Read the model definition and answer for the solid it produces. Units are mm, in the model's axes. A direction names the side the tool comes from. Give positions to 0.01 mm unless a question says otherwise; leave off trailing zeros. Loops run counter-clockwise (first coordinate to the right, second up) from the corner with the lowest first, then second, coordinate; pieces in that order, holes last.
(1) Which of the six approach directions +Z, -Z, +X, -X, +Y, -Y give full straight-line access (tool end or side, diameter ignored) to faces 5 (the face through (28, -8, 2)), 6 (the face through (-17.034, -7.348, 9.691)), 7 (the face through (29, -29.583, 10))?
(2) Determine the mould class of faces 1 (the face through (66.391, 25.125, 9.691)), 2 (the face through (29, 26.842, 10)), 3 (the face through (20.6, -31.9, 17.6)), 4 (the face through (40.956, -36.022, 9.691)) for opening direction Y: pulls with the +Y half, pulls with the -Y half, needs draft (parallel to the pull), parting line crosses it, or undercut.
(3) Each of these flat-tipped pins is pushed along its axis until it touches: P1, Ø1.5, axis at y = -30, z = 10, coming from the +X side (3 decimals); P2, Ø4.5, axis at x = -3.5, y = -38, coming from the +Z side; P3, Ø0.8, axis at x = 31, y = -29, coming from the +Z side; P4, Ø3, axis at x = 50, z = 3, coming from the -Y side. Where does it stop, or does it pass through?
(4) Straight lines are drawn through the part: probe 1 along Y at (x, z) = (55, 17.25); probe 2 along X at (y, z) = (-1, 9.5); probe 3 along X at (y, z) = (1, 9.25). For each, find the intervals that lie inside material, in ascending order.
(5) Find section B-B, the plane z = 11.75. State how many separate pieces and enclosed holes the cut face has, then the cut area to 3 significant figures.
(6) Find section A-A, the plane x = 29. Write down the section's boundary in (y, z).
```python
from build123d import *

# Parameters (mm, degrees)
EXTRUDE_1_DEPTH                    = 2
EXTRUDE_2_DEPTH                    = 14
EXTRUDE_3_DEPTH                    = 15.6000508
FILLET_1_R                         = 2
SKETCH_12_W                        = 10.2
SKETCH_12_H                        = 1.9
USB_TYPEC_LOWER_HALF_OPENING_DEPTH = 4


with BuildPart() as part:
    # 草图1 → 凸台-拉伸1 (new body)
    with BuildSketch(Plane.XY):
        with BuildLine():
            Line((-18.736989068, -43.807492656), (7.319785463, -43.807492656))
            ThreePointArc((7.319785463, -43.807492656), (8.845661337, -43.503976443), (10.139236063, -42.639636403))
            Line((10.139236063, -42.639636403), (23.19168867, -29.587186336))
            ThreePointArc((23.19168867, -29.587186336), (23.195810689, -29.58443157), (23.200673199, -29.583464208))
            Line((23.200673199, -29.583464208), (34.512272144, -29.583464208))
            ThreePointArc((34.512272144, -29.583464208), (34.51713329, -29.584431533), (34.521254362, -29.587185298))
            Line((34.521254362, -29.587185298), (47.573709045, -42.639637441))
            ThreePointArc((47.573709045, -42.639637441), (48.867282822, -43.503976481), (50.393157333, -43.807492656))
            Line((50.393157333, -43.807492656), (75.552353414, -43.807492656))
            ThreePointArc((75.552353414, -43.807492656), (78.607819066, -42.38196989), (79.478533005, -39.124694535))
            Line((79.478533005, -39.124694535), (68.376081771, 23.550429382))
            ThreePointArc((68.376081771, 23.550429382), (67.011684276, 25.910401612), (64.449902577, 26.842240644))
            Line((64.449902577, 26.842240644), (-7.634537883, 26.842240644))
            ThreePointArc((-7.634537883, 26.842240644), (-10.196320099, 25.910401179), (-11.560717313, 23.550428053))
            Line((-11.560717313, 23.550428053), (-22.663168183, -39.124693813))
            ThreePointArc((-22.663168183, -39.124693813), (-21.792454719, -42.381969476), (-18.736989068, -43.807492656))
        make_face()
    extrude(amount=EXTRUDE_1_DEPTH)

    # 草图4 → 凸台-拉伸2 (add)
    # profile 1 of 4: a face of its own
    with BuildSketch(Plane.XY.offset(2)):
        with BuildLine():
            ThreePointArc((-5.872384963, -37.375183791), (-2.822381153, -40.425187601), (0.227622657, -37.375183791))
            ThreePointArc((0.227622657, -37.375183791), (-2.822381153, -34.325179981), (-5.872384963, -37.375183791))
        make_face()
        with BuildLine():
            ThreePointArc((-0.772377343, -37.375183791), (-2.822381153, -35.325179981), (-4.872384963, -37.375183791))
            ThreePointArc((-4.872384963, -37.375183791), (-2.822381153, -39.425187601), (-0.772377343, -37.375183791))
        make_face(mode=Mode.SUBTRACT)
    # profile 2 of 4: a face of its own
    with BuildSketch(Plane.XY.offset(2)):
        with BuildLine():
            ThreePointArc((56.727742037, -37.375183791), (59.777745847, -40.425187601), (62.827749657, -37.375183791))
            ThreePointArc((62.827749657, -37.375183791), (59.777745847, -34.325179981), (56.727742037, -37.375183791))
        make_face()
        with BuildLine():
            ThreePointArc((61.827749657, -37.375183791), (59.777745847, -35.325179981), (57.727742037, -37.375183791))
            ThreePointArc((57.727742037, -37.375183791), (59.777745847, -39.425187601), (61.827749657, -37.375183791))
        make_face(mode=Mode.SUBTRACT)
    # profile 3 of 4: a face of its own
    with BuildSketch(Plane.XY.offset(2)):
        with BuildLine():
            ThreePointArc((69.049761341, 9.106909173), (65.999757531, 12.156912983), (62.949753721, 9.106909173))
            ThreePointArc((62.949753721, 9.106909173), (65.999757531, 6.056905363), (69.049761341, 9.106909173))
        make_face()
        with BuildLine():
            ThreePointArc((63.949753721, 9.106909173), (65.999757531, 7.056905363), (68.049761341, 9.106909173))
            ThreePointArc((68.049761341, 9.106909173), (65.999757531, 11.156912983), (63.949753721, 9.106909173))
        make_face(mode=Mode.SUBTRACT)
    # profile 4 of 4: a face of its own
    with BuildSketch(Plane.XY.offset(2)):
        with BuildLine():
            ThreePointArc((-6.519385217, 1.613894187), (-3.469381407, -1.436109623), (-0.419377597, 1.613894187))
            ThreePointArc((-0.419377597, 1.613894187), (-3.469381407, 4.663897997), (-6.519385217, 1.613894187))
        make_face()
        with BuildLine():
            ThreePointArc((-1.419377597, 1.613894187), (-3.469381407, 3.663897997), (-5.519385217, 1.613894187))
            ThreePointArc((-5.519385217, 1.613894187), (-3.469381407, -0.436109623), (-1.419377597, 1.613894187))
        make_face(mode=Mode.SUBTRACT)
    extrude(amount=EXTRUDE_2_DEPTH)

    # 草图6 → 凸台-拉伸3 (add)
    with BuildSketch(Plane.XY.offset(2)):
        with BuildLine():
            Line((-11.560717313, 23.550428053), (-22.663168183, -39.124693813))
            ThreePointArc((-22.663168183, -39.124693813), (-21.792454719, -42.381969476), (-18.736989068, -43.807492656))
            Line((-18.736989068, -43.807492656), (7.319785463, -43.807492656))
            ThreePointArc((7.319785463, -43.807492656), (8.845661337, -43.503976443), (10.139236063, -42.639636403))
            Line((10.139236063, -42.639636403), (23.19168867, -29.587186337))
            ThreePointArc((23.19168867, -29.587186337), (23.195810689, -29.58443157), (23.200673199, -29.583464208))
            Line((23.200673199, -29.583464208), (34.512272144, -29.583464208))
            ThreePointArc((34.512272144, -29.583464208), (34.51713329, -29.584431533), (34.521254362, -29.587185298))
            Line((34.521254362, -29.587185298), (47.573709045, -42.639637441))
            ThreePointArc((47.573709045, -42.639637441), (48.867282822, -43.503976481), (50.393157333, -43.807492656))
            Line((50.393157333, -43.807492656), (75.552353414, -43.807492656))
            ThreePointArc((75.552353414, -43.807492656), (78.607819066, -42.38196989), (79.478533005, -39.124694535))
            Line((79.478533005, -39.124694535), (68.376081771, 23.550429382))
            ThreePointArc((68.376081771, 23.550429382), (67.011684276, 25.910401612), (64.449902577, 26.842240644))
            Line((64.449902577, 26.842240644), (-7.634537883, 26.842240644))
            ThreePointArc((-7.634537883, 26.842240644), (-10.196320099, 25.910401179), (-11.560717313, 23.550428053))
        make_face()
        with BuildLine():
            Line((-10.576047254, 23.376000774), (-21.678498124, -39.299121091))
            ThreePointArc((-21.678498124, -39.299121091), (-21.026156001, -41.739485021), (-18.736988894, -42.807492656))
            Line((-18.736988894, -42.807492656), (7.319785463, -42.807492656))
            ThreePointArc((7.319785463, -42.807492656), (8.462977611, -42.580097033), (9.432128831, -41.932530072))
            Line((9.432128831, -41.932530072), (22.484540842, -28.880120606))
            ThreePointArc((22.484540842, -28.880120606), (22.813100147, -28.660563268), (23.200672562, -28.583464208))
            Line((23.200672562, -28.583464208), (34.512322586, -28.58346421))
            ThreePointArc((34.512322586, -28.58346421), (34.899840317, -28.660561774), (35.228361593, -28.880078967))
            Line((35.228361593, -28.880078967), (48.280815757, -41.932530591))
            ThreePointArc((48.280815757, -41.932530591), (49.249966503, -42.580097051), (50.393157969, -42.807492656))
            Line((50.393157969, -42.807492656), (75.552353414, -42.807492656))
            ThreePointArc((75.552353414, -42.807492656), (77.841520522, -41.739485228), (78.493862882, -39.299121453))
            Line((78.493862882, -39.299121453), (67.391411713, 23.376002103))
            ThreePointArc((67.391411713, 23.376002103), (66.369199703, 25.144102993), (64.449902443, 25.842240644))
            Line((64.449902443, 25.842240644), (-7.634537883, 25.842240644))
            ThreePointArc((-7.634537883, 25.842240644), (-9.553835577, 25.144102517), (-10.576047254, 23.376000774))
        make_face(mode=Mode.SUBTRACT)
    extrude(amount=EXTRUDE_3_DEPTH)

    # 圆角1
    fillet_1_edges = [part.edges().sort_by_distance(p)[0] for p in [
        (28.407682347, 26.842240644, 0),
        (67.011684276, 25.910401612, 0),
        (73.927307388, -7.787132577, 0),
        (78.607819066, -42.38196989, 0),
        (62.972755373, -43.807492656, 0),
        (48.867282822, -43.503976481, 0),
        (41.047481703, -36.11341137, 0),
        (34.51713329, -29.584431533, 0),
        (28.856472671, -29.583464208, 0),
        (23.195810689, -29.58443157, 0),
        (16.665462366, -36.11341137, 0),
        (8.845661337, -43.503976443, 0),
        (-5.708601803, -43.807492656, 0),
        (-21.792454719, -42.381969476, 0),
        (-17.111942748, -7.78713288, 0),
        (-10.196320099, 25.910401179, 0),
    ]]
    fillet(fillet_1_edges, radius=FILLET_1_R - 0.0001)  # a hair under: the kernel refuses the full size

    # 草图12 → USB_TypeC_Lower_Half_Opening (cut)
    with BuildSketch(Plane.XZ.offset(29.583464208)):
        with Locations((28.634, 17.05)):
            Rectangle(SKETCH_12_W, SKETCH_12_H)
    extrude(amount=-USB_TYPEC_LOWER_HALF_OPENING_DEPTH, mode=Mode.SUBTRACT)


solid = part.part
```
Entries:
1. face 5: +Z
1. face 6: +Z, -Z, -X, +Y
1. face 7: +Z, -Z, -Y
2. face 1: undercut
2. face 2: pulls with the +Y half
2. face 3: needs draft
2. face 4: pulls with the -Y half
3. P1: stops at x = 77.995
3. P2: stops at z = 16
3. P3: stops at z = 16.1
3. P4: stops at y = -43.81
4. probe 1: y = -43.81 to -42.81, 25.84 to 26.84
4. probe 2: x = -15.91 to -14.89, -5.04 to -1.9, 71.71 to 72.73
4. probe 3: x = -15.56 to -14.54, -6.46 to -5.43, -1.51 to -0.48, 71.36 to 72.37
5. separate pieces: 5
5. enclosed holes: 5
5. area: 391 mm2
6. outline: (-29.58, 2) arc R2 ccw to (-27.58, 0) - (24.84, 0) arc R2 ccw to (26.84, 2) - (26.84, 17.6) - (25.84, 17.6) - (25.84, 2) - (-28.58, 2) - (-28.58, 16.1) - (-29.58, 16.1) - close
